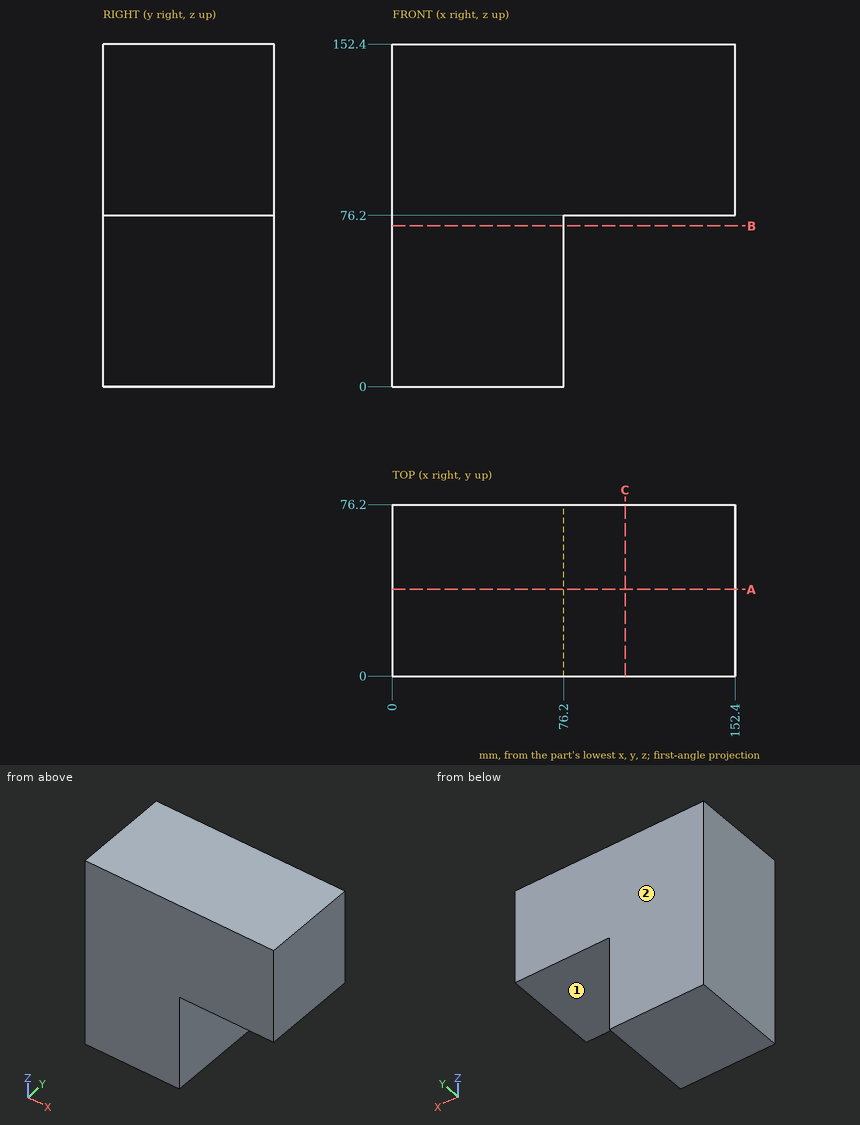
Geometry check sheet. Reference: drawing and pictorial views, mm from the part's lowest x, y, z. A direction names the side the tool comes from. Coordinates: 2 decimals unless noted, no trailing zeros. Loops run counter-clockwise (first coordinate to the right, second up) from the corner with the lowest first, then second, coordinate; pieces in that order, holes last.
1) Sectioned sample at B-B (z = 71.5). Record the boundary of the cut face in (x, y).
2) Access from +Z, -Z, +X, -X, +Y, -Y to the whole of each face (thin tool, end or side, straight path). Record for the marked faces 1 and 2.
3) Sectioned sample at A-A (y = 38.5). Record the boundary of the cut face in (x, z), and give its area (3 significant figures).
4) Sectioned sample at C-C (x = 103.5). Record the boundary of the cut face in (y, z).
5) Material ranges on probe 1 along X at (y, z) = (15.5, 36.5); probe 2 along Z at (x, y) = (86, 60), recorded low to high.
Check sheet entries:
1. outline: (0, 0) - (76.2, 0) - (76.2, 76.2) - (0, 76.2) - close
2. face 1: -Z, +X, +Y, -Y
2. face 2: +Z, -Z, +X, -X, +Y
3. outline: (0, 0) - (76.2, 0) - (76.2, 76.2) - (152.4, 76.2) - (152.4, 152.4) - (0, 152.4) - close
3. area: 17,400 mm2
4. outline: (0, 76.2) - (76.2, 76.2) - (76.2, 152.4) - (0, 152.4) - close
5. probe 1: x = 0 to 76.2
5. probe 2: z = 76.2 to 152.4
